Work out the finished part from the listing and answer in its coordinate system (mm). Face numbers are marked on the shaded views. A direction names the side the tool comes from. Give positions to 0.01 mm unless a question says otherwise; leave off trailing zeros. Write each loop counter-clockwise with the first axis right and the second up, starting at its lowest first coordinate (ties: lowest second). Pieces come first, ordered by that corner, then holes. Notation, with made-up numbers: (85.25, -17.75) - (118.25, -17.75) arc R35 cw to (118.25, 20.25) - close; hole circle Ø4 at (22.25, 2). An arc over 180 degrees is marked (long way). Write item = value, one per line.
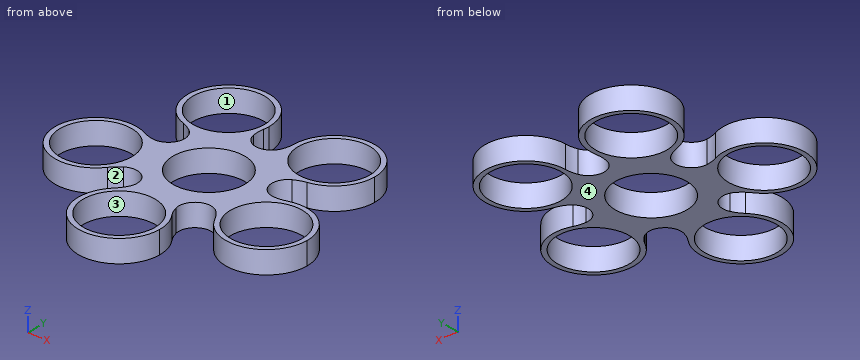
from build123d import *

# Parameters (mm, degrees)
F0_R     = 11.25
F1_DEPTH = 7
F2_R     = 5.08


# Not quite as in the source:
# - a feature names something its author has since deleted; it is built from what else it names


with BuildPart() as f1:
    # F0 (on Top) → F1 (new body)
    with BuildSketch(Plane.XY):
        with BuildLine():
            ThreePointArc((-10.2261463935, 7.6719560941), (-6.6075524932, 10.9440956877), (-2.0266855863, 12.6224215548))
            ThreePointArc((-2.0266855863, 12.6224215548), (-0.3918821811, 13.0140427744), (1.1648785444, 13.648428617))
            ThreePointArc((1.1648785444, 13.648428617), (-2.5221716271, 18.3553828089), (-3.2272094242, 24.2927794132))
            ThreePointArc((-3.2272094242, 24.2927794132), (-9.2505734905, 15.3217339628), (-19.9945367973, 14.1694216731))
            ThreePointArc((-19.9945367973, 14.1694216731), (-15.0686816006, 10.7803646784), (-12.6204597068, 5.3254617195))
            ThreePointArc((-12.6204597068, 5.3254617195), (-11.3340606288, 6.4076478244), (-10.2261463935, 7.6719560941))
        make_face()
        with BuildLine():
            ThreePointArc((12.7825888677, -0.1959648224), (12.7837153932, -0.0979852894), (12.7840909091, 0))
            ThreePointArc((12.7840909091, 0), (12.4276891989, 2.9975859532), (11.3783559826, 5.828035304))
            ThreePointArc((11.3783559826, 5.828035304), (8.3666075071, 9.666067411), (4.1364108135, 12.0964079773))
            ThreePointArc((4.1364108135, 12.0964079773), (1.0871557866, 12.7377813087), (-2.0266855863, 12.6224215548))
            ThreePointArc((-2.0266855863, 12.6224215548), (-6.6075524932, 10.9440956877), (-10.2261463935, 7.6719560941))
            ThreePointArc((-10.2261463935, 7.6719560941), (-11.7784003031, 4.9701374901), (-12.6309165595, 1.9730502372))
            ThreePointArc((-12.6309165595, 1.9730502372), (-12.4502995304, -2.9022442999), (-10.4565168586, -7.3548783509))
            ThreePointArc((-10.4565168586, -7.3548783509), (-8.3666075071, -9.666067411), (-5.7796501565, -11.4030094467))
            ThreePointArc((-5.7796501565, -11.4030094467), (-1.0871557866, -12.7377813087), (3.7636635709, -12.2175208981))
            ThreePointArc((3.7636635709, -12.2175208981), (6.6075524932, -10.9440956877), (9.0588963197, -9.0204976493))
            ThreePointArc((9.0588963197, -9.0204976493), (11.7784003031, -4.9701374901), (12.7825888677, -0.1959648224))
        make_face()
        Circle(F0_R, mode=Mode.SUBTRACT)
        with BuildLine():
            ThreePointArc((-2.0266855863, 12.6224215548), (1.0871557866, 12.7377813087), (4.1364108135, 12.0964079773))
            ThreePointArc((4.1364108135, 12.0964079773), (2.591617868, 12.7594042888), (1.1648785444, 13.648428617))
            ThreePointArc((1.1648785444, 13.648428617), (-0.3918821811, 13.0140427744), (-2.0266855863, 12.6224215548))
        make_face()
        with BuildLine():
            ThreePointArc((11.3783559826, 5.828035304), (12.4276891989, 2.9975859532), (12.7840909091, 0))
            ThreePointArc((12.7840909091, 0), (12.7837153932, -0.0979852894), (12.7825888677, -0.1959648224))
            ThreePointArc((12.7825888677, -0.1959648224), (12.935768557, 1.4780977023), (13.34039424, 3.1097310588))
            ThreePointArc((13.34039424, 3.1097310588), (12.2559919302, 4.3942624848), (11.3783559826, 5.828035304))
        make_face()
        with BuildLine():
            ThreePointArc((-12.6309165595, 1.9730502372), (-11.7784003031, 4.9701374901), (-10.2261463935, 7.6719560941))
            ThreePointArc((-10.2261463935, 7.6719560941), (-11.3340606288, 6.4076478244), (-12.6204597068, 5.3254617195))
            ThreePointArc((-12.6204597068, 5.3254617195), (-12.4981884377, 3.6488582809), (-12.6309165595, 1.9730502372))
        make_face()
        with BuildLine():
            ThreePointArc((-10.4565168586, -7.3548783509), (-12.4502995304, -2.9022442999), (-12.6309165595, 1.9730502372))
            ThreePointArc((-12.6309165595, 1.9730502372), (-12.4981884377, 3.6488582809), (-12.6204597068, 5.3254617195))
            ThreePointArc((-12.6204597068, 5.3254617195), (-18.236400325, 3.273397465), (-24.1010687164, 4.4376231269))
            ThreePointArc((-24.1010687164, 4.4376231269), (-18.9875890794, -0.2741455025), (-17.0966279638, -6.9653863197))
            ThreePointArc((-17.0966279638, -6.9653863197), (-17.7529621653, -11.0089611755), (-19.6545724794, -14.6373424139))
            ThreePointArc((-19.6545724794, -14.6373424139), (-14.9092147728, -10.999851937), (-8.9647515968, -10.3571122686))
            ThreePointArc((-8.9647515968, -10.3571122686), (-9.5964525671, -8.7992601454), (-10.4565168586, -7.3548783509))
        make_face()
        with BuildLine():
            ThreePointArc((4.1364108135, 12.0964079773), (8.3666075071, 9.666067411), (11.3783559826, 5.828035304))
            ThreePointArc((11.3783559826, 5.828035304), (12.2559919302, 4.3942624848), (13.34039424, 3.1097310588))
            ThreePointArc((13.34039424, 3.1097310588), (16.677612534, 8.0708529874), (22.1065436034, 10.5761402317))
            ThreePointArc((22.1065436034, 10.5761402317), (11.7132505099, 13.5324943754), (7.2972691493, 23.3945266088))
            ThreePointArc((7.2972691493, 23.3945266088), (5.596257378, 17.6624837194), (1.1648785444, 13.648428617))
            ThreePointArc((1.1648785444, 13.648428617), (2.591617868, 12.7594042888), (4.1364108135, 12.0964079773))
        make_face()
        with BuildLine():
            ThreePointArc((13.34039424, 3.1097310588), (12.935768557, 1.4780977023), (12.7825888677, -0.1959648224))
            ThreePointArc((12.7825888677, -0.1959648224), (11.7784003031, -4.9701374901), (9.0588963197, -9.0204976493))
            ThreePointArc((9.0588963197, -9.0204976493), (7.9665017598, -10.2982392034), (7.0799385192, -11.7265091268))
            ThreePointArc((7.0799385192, -11.7265091268), (12.8295030243, -13.3673213445), (16.8898047449, -17.7563652803))
            ThreePointArc((16.8898047449, -17.7563652803), (16.4897604244, -6.9581924862), (24.5044971566, 0.2891909218))
            ThreePointArc((24.5044971566, 0.2891909218), (18.52735887, 0.1356505859), (13.34039424, 3.1097310588))
        make_face()
        with BuildLine():
            ThreePointArc((7.0799385192, -11.7265091268), (7.9665017598, -10.2982392034), (9.0588963197, -9.0204976493))
            ThreePointArc((9.0588963197, -9.0204976493), (6.6075524932, -10.9440956877), (3.7636635709, -12.2175208981))
            ThreePointArc((3.7636635709, -12.2175208981), (5.4031267709, -11.8458896701), (7.0799385192, -11.7265091268))
        make_face()
        with BuildLine():
            ThreePointArc((-8.9647515968, -10.3571122686), (-7.3324230712, -10.7589243367), (-5.7796501565, -11.4030094467))
            ThreePointArc((-5.7796501565, -11.4030094467), (-8.3666075071, -9.666067411), (-10.4565168586, -7.3548783509))
            ThreePointArc((-10.4565168586, -7.3548783509), (-9.5964525671, -8.7992601454), (-8.9647515968, -10.3571122686))
        make_face()
        with BuildLine():
            ThreePointArc((7.0799385192, -11.7265091268), (5.4031267709, -11.8458896701), (3.7636635709, -12.2175208981))
            ThreePointArc((3.7636635709, -12.2175208981), (-1.0871557866, -12.7377813087), (-5.7796501565, -11.4030094467))
            ThreePointArc((-5.7796501565, -11.4030094467), (-7.3324230712, -10.7589243367), (-8.9647515968, -10.3571122686))
            ThreePointArc((-8.9647515968, -10.3571122686), (-8.7485436062, -16.3323119169), (-11.6680702077, -21.5501774915))
            ThreePointArc((-11.6680702077, -21.5501774915), (-1.5220181013, -17.8328938321), (7.8473429707, -23.2157967899))
            ThreePointArc((7.8473429707, -23.2157967899), (5.8542801254, -17.5786470467), (7.0799385192, -11.7265091268))
        make_face()
        with BuildLine():
            ThreePointArc((41.0522516366, -11.9283299763), (35.8615118695, -1.64368128), (24.5044971566, 0.2891909218))
            ThreePointArc((24.5044971566, 0.2891909218), (16.4897604244, -6.9581924862), (16.8898047449, -17.7563652803))
            ThreePointArc((16.8898047449, -17.7563652803), (31.2657466808, -24.3560191752), (41.0522516366, -11.9283299763))
        make_face()
        with Locations((28.2681607275, -11.9283299763)):
            Circle(F0_R, mode=Mode.SUBTRACT)
        with BuildLine():
            ThreePointArc((10.1749170211, -30.5706751408), (9.5791410589, -26.713479381), (7.8473429707, -23.2157967899))
            ThreePointArc((7.8473429707, -23.2157967899), (-1.5220181013, -17.8328938321), (-11.6680702077, -21.5501774915))
            ThreePointArc((-11.6680702077, -21.5501774915), (-7.4888883409, -42.3868237193), (10.1749170211, -30.5706751408))
        make_face()
        with Locations((-2.6091738879, -30.5706751408)):
            Circle(F0_R, mode=Mode.SUBTRACT)
        with BuildLine():
            ThreePointArc((-17.0966279638, -6.9653863197), (-18.9875890794, -0.2741455025), (-24.1010687164, 4.4376231269))
            ThreePointArc((-24.1010687164, 4.4376231269), (-42.3310184032, -9.8676306196), (-19.6545724794, -14.6373424139))
            ThreePointArc((-19.6545724794, -14.6373424139), (-17.7529621653, -11.0089611755), (-17.0966279638, -6.9653863197))
        make_face()
        with Locations((-29.8807188729, -6.9653863197)):
            Circle(F0_R, mode=Mode.SUBTRACT)
        with BuildLine():
            ThreePointArc((-19.9945367973, 14.1694216731), (-9.2505734905, 15.3217339628), (-3.2272094242, 24.2927794132))
            ThreePointArc((-3.2272094242, 24.2927794132), (-3.112386187, 25.2763361411), (-3.0740350747, 26.2658296504))
            ThreePointArc((-3.0740350747, 26.2658296504), (-23.2929335971, 36.6656669628), (-19.9945367973, 14.1694216731))
        make_face()
        with Locations((-15.8581259838, 26.2658296504)):
            Circle(F0_R, mode=Mode.SUBTRACT)
        with BuildLine():
            ThreePointArc((7.2972691493, 23.3945266088), (11.7132505099, 13.5324943754), (22.1065436034, 10.5761402317))
            ThreePointArc((22.1065436034, 10.5761402317), (29.8097684265, 14.9062868395), (32.8639489261, 23.1985617864))
            ThreePointArc((32.8639489261, 23.1985617864), (20.1778433064, 35.9822771796), (7.2972691493, 23.3945266088))
        make_face()
        with Locations((20.079858017, 23.1985617864)):
            Circle(F0_R, mode=Mode.SUBTRACT)
    extrude(amount=F1_DEPTH)

    # F2
    f2_edges = [f1.edges().sort_by_distance(p)[0] for p in [
        (7.079939, -11.726509, 3.5),
        (-8.964752, -10.357112, 3.5),
        (-12.62046, 5.325462, 3.5),
        (1.164879, 13.648429, 3.5),
        (13.340394, 3.109731, 3.5),
    ]]
    fillet(f2_edges, radius=F2_R)


solid = f1.part
1. A tool of negligible diameter and unlimited length cuts with its end or side. For the marked faces 1 and 2, from which of +Z, -Z, +X, -X, +Y, -Y can it reach the whole face along a straight path? Write none if from no direction.
Solution:
face_1 = +Z, -Z
face_2 = +Z, -Z, -Y
2. Given pin 1 (3 mm diameter, centred on x = -26.5, z = 4.5, fed in from -Y), flat-ended and moving along its own axis, determine where the tip first touches the part or whether it passes through.
Solution:
pin_1 = -19.61
3. Straight lines are drawn through the part: line 1 (Y direction, x = 22, z = 1); line 2 (X direction, y = -9.5, z = 1); line 3 (X direction, y = -30, z = 5.25). For each, find the intervals that lie inside material, in ascending order.
Solution:
line_1 = -23.07 to -21.27, -2.59 to -0.18, 10.56 to 12.11, 34.28 to 35.84
line_2 = -42.41 to -40.84, -18.92 to -6.03, 6.03 to 17.28, 39.25 to 40.82
line_3 = -15.38 to -13.84, 8.63 to 10.16
4. Find section B-B, the plane x = 0. Give the number of separate pieces and of enclosed holes in the cut face, then the cut area to 3 significant figures.
Solution:
separate_pieces = 3
enclosed_holes = 0
area = 108 mm^2
5. For a pull along X with two mould halves and no side action, classify the marked faces 3 and 4 as pulls with the +X half, pulls with the -X half, needs draft (parallel to the pull), parting line crosses it, or undercut.
Solution:
face_3 = undercut
face_4 = needs draft
6. Find section A-A, the plane y = -29.5. Give the vertices of the cut face in (x, z).
Solution:
outline = (-15.35, 0) - (-13.81, 0) - (-13.81, 7) - (-15.35, 7) - close; (8.59, 0) - (10.13, 0) - (10.13, 7) - (8.59, 7) - close
